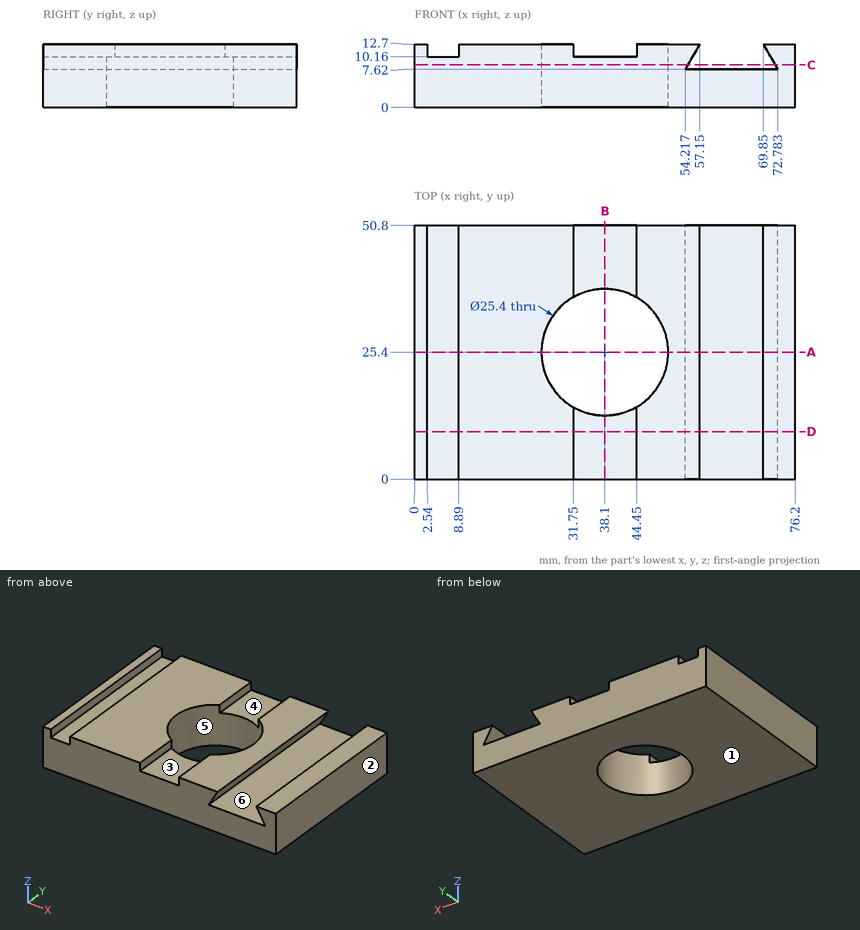
Here's the drawing with two shaded views (mm, measured from the low corner). I have some questions. A direction names the side the tool comes from. Round coordinates to 2 decimals unless told otherwise and drop trailing zeros. Loops run counter-clockwise (first coordinate to the right, second up) from the corner with the lowest first, then second, coordinate; pieces in that order, holes last.
1. Suppose I cut it at C-C, the plane z = 8.5. Please give me the cut outline in (x, y) (3 decimals), and give its area (3 significant figures).
Answers:
outline: (0, 0) - (54.725, 0) - (54.725, 50.8) - (0, 50.8) - close; (72.275, 0) - (76.2, 0) - (76.2, 50.8) - (72.275, 50.8) - close; hole circle Ø25.4 at (38.1, 25.4)
area: 2,470 mm2
2. Suppose I cut it at B-B, the plane x = 38.1. Please give me the cut outline in (y, z).
Answers:
outline: (0, 0) - (12.7, 0) - (12.7, 10.16) - (0, 10.16) - close; (38.1, 0) - (50.8, 0) - (50.8, 10.16) - (38.1, 10.16) - close
3. For the marked faces 4, 5 and 6, which set-ups out of +Z, -Z, +X, -X, +Y, -Y let a thin tool reach every point of the face, with its end or its side?
Answers:
face 4: +Z, +Y, -Y
face 5: +Z, -Z
face 6: +Y, -Y
4. If I drill on probe 1 along Y at (x, z) = (38.1, 4.5); probe 2 along X at (y, z) = (25.4, 5.25); probe 3 along X at (y, z) = (25.4, 10), over which ranges is the centre line in solid material (lowest first)?
Answers:
probe 1: y = 0 to 12.7, 38.1 to 50.8
probe 2: x = 0 to 25.4, 50.8 to 76.2
probe 3: x = 0 to 25.4, 50.8 to 55.59, 71.41 to 76.2
5. Thinking about a two-plate mould opening in X: for the marked faces 1, 2 and 3, which applies, released by +X, released by -X, zero draft, split by the parting line, or undercut?
Answers:
face 1: zero draft
face 2: released by +X
face 3: undercut
6. Will these pins go through, and if not, where does the flat tip stop? pin 1 (5.5 mm diameter, centred on x = 65, y = 33, fed in from +Z); pin 2 (4 mm diameter, centred on x = 39, y = 47, fed in from +Z).
Answers:
pin 1: stops at z = 7.62
pin 2: stops at z = 10.16
7. Suppose I cut it at D-D, the plane y = 9.5. Please give me the cut outline in (x, z).
Answers:
outline: (0, 0) - (76.2, 0) - (76.2, 12.7) - (69.85, 12.7) - (72.78, 7.62) - (54.22, 7.62) - (57.15, 12.7) - (44.45, 12.7) - (44.45, 10.16) - (31.75, 10.16) - (31.75, 12.7) - (8.89, 12.7) - (8.89, 10.16) - (2.54, 10.16) - (2.54, 12.7) - (0, 12.7) - close
8. Suppose I cut it at A-A, the plane y = 25.4. Please give me the cut outline in (x, z).
Answers:
outline: (0, 0) - (25.4, 0) - (25.4, 12.7) - (8.89, 12.7) - (8.89, 10.16) - (2.54, 10.16) - (2.54, 12.7) - (0, 12.7) - close; (50.8, 0) - (76.2, 0) - (76.2, 12.7) - (69.85, 12.7) - (72.78, 7.62) - (54.22, 7.62) - (57.15, 12.7) - (50.8, 12.7) - close
